```python
from build123d import *

# Parameters (mm, degrees)
SKETCH1_W           = 75
SKETCH1_H           = 85
BOSS_EXTRUDE1_DEPTH = 3
SKETCH2_R           = 2.5
BOSS_EXTRUDE2_DEPTH = 2
SKETCH3_R           = 0.75
BOSS_EXTRUDE3_DEPTH = 4
CUT_EXTRUDE1_REACH  = 58.996
CHAMFER3_SIZE       = 2.5
FILLET2_R           = 1
SKETCH5_W           = 9.85
SKETCH5_H           = 3.85
BOSS_EXTRUDE4_DEPTH = 3
FILLET3_R           = 2
SKETCH6_W           = 1.5
SKETCH6_H           = 3
CUT_EXTRUDE2_DEPTH  = 69.085465593


with BuildPart() as part:
    # Sketch1 → Boss-Extrude1 (new body)
    with BuildSketch(Plane(origin=(0, 0, 0), x_dir=(1, 0, 0), z_dir=(0, 1, 0))):
        Rectangle(SKETCH1_W, SKETCH1_H)
    extrude(amount=BOSS_EXTRUDE1_DEPTH)

    # Sketch2 → Boss-Extrude2 (add)
    with BuildSketch(Plane(origin=(0, 3, 0), x_dir=(1, 0, 0), z_dir=(0, 1, 0))):
        with Locations(Location((27.93, 36.82, 0), (0, 0, 270))):
            Circle(SKETCH2_R)
        with Locations(Location((27.93, 17.77, 0), (0, 0, 270))):
            Circle(SKETCH2_R)
        with Locations(Location((-27.93, 17.77, 0), (0, 0, 90))):
            Circle(SKETCH2_R)
        with Locations(Location((-27.93, 36.82, 0), (0, 0, 90))):
            Circle(SKETCH2_R)
        with Locations(Location((-19.05, 10.79, 0), (0, 0, 90))):
            Circle(SKETCH2_R)
        with Locations(Location((-20.32, -37.48, 0), (0, 0, 90))):
            Circle(SKETCH2_R)
        with Locations(Location((31.75, -4.45, 0), (0, 0, 270))):
            Circle(SKETCH2_R)
        with Locations(Location((31.75, -32.4, 0), (0, 0, 270))):
            Circle(SKETCH2_R)
    extrude(amount=BOSS_EXTRUDE2_DEPTH)

    # Sketch3 → Boss-Extrude3 (add)
    with BuildSketch(Plane(origin=(0, 5, 0), x_dir=(1, 0, 0), z_dir=(0, 1, 0))):
        with Locations(Location((-27.93, 36.82, 0), (0, 0, 270))):
            Circle(SKETCH3_R)
        with Locations(Location((27.93, 36.82, 0), (0, 0, 90))):
            Circle(SKETCH3_R)
        with Locations(Location((27.93, 17.77, 0), (0, 0, 270))):
            Circle(SKETCH3_R)
        with Locations(Location((-27.93, 17.77, 0), (0, 0, 90))):
            Circle(SKETCH3_R)
        with Locations(Location((-19.05, 10.79, 0), (0, 0, 270))):
            Circle(SKETCH3_R)
        with Locations(Location((31.75, -4.45, 0), (0, 0, 270))):
            Circle(SKETCH3_R)
        with Locations(Location((-20.32, -37.48, 0), (0, 0, 270))):
            Circle(SKETCH3_R)
        with Locations(Location((31.75, -32.4, 0), (0, 0, 270))):
            Circle(SKETCH3_R)
    extrude(amount=BOSS_EXTRUDE3_DEPTH)

    # Sketch4 → Cut-Extrude1 (cut, up to next)
    with BuildSketch(Plane(origin=(0, 3, 0), x_dir=(1, 0, 0), z_dir=(0, 1, 0)), mode=Mode.PRIVATE) as cut_extrude1_sk1:
        Polygon((37.5, 7.5), (32.5, 12.5), (32.5, 42.5), (37.5, 42.5), align=None)
    cut_extrude1_tool1 = extrude(cut_extrude1_sk1.sketch, amount=-CUT_EXTRUDE1_REACH, mode=Mode.PRIVATE) & part.part
    add(cut_extrude1_tool1.solids().sort_by_distance((35.064103, 3, -26.217949))[0], mode=Mode.SUBTRACT)

    # Chamfer3
    chamfer3_edges = [part.edges().sort_by_distance(p)[0] for p in [
        (37.5, 1.5, 42.5),
        (-37.5, 1.5, 42.5),
        (-37.5, 1.5, -42.5),
        (32.5, 1.5, -42.5),
    ]]
    chamfer(chamfer3_edges, length=CHAMFER3_SIZE)

    # Fillet2
    fillet2_edges = [part.edges().sort_by_distance(p)[0] for p in [
        (-37.5, 1.5, -40),
        (-37.5, 1.5, 40),
        (37.5, 1.5, 40),
        (32.5, 1.5, -40),
        (-35, 1.5, -42.5),
        (30, 1.5, -42.5),
        (37.5, 1.5, -7.5),
        (32.5, 1.5, -12.5),
        (35, 1.5, 42.5),
        (-35, 1.5, 42.5),
    ]]
    fillet(fillet2_edges, radius=FILLET2_R)

    # Sketch5 → Boss-Extrude4 (add)
    with BuildSketch(Plane.XZ):
        with Locations((10, -9.0625)):
            Rectangle(SKETCH5_W, SKETCH5_H)
        with Locations((-10, -9.0625)):
            Rectangle(SKETCH5_W, SKETCH5_H)
    extrude(amount=BOSS_EXTRUDE4_DEPTH)

    # Fillet3
    fillet3_edges = [part.edges().sort_by_distance(p)[0] for p in [
        (10, 0, -7.1375),
        (10, 0, -10.9875),
        (-10, 0, -10.9875),
        (-10, 0, -7.1375),
    ]]
    fillet(fillet3_edges, radius=FILLET3_R)

    # Sketch6 → Cut-Extrude2 (cut, through all)
    with BuildSketch(Plane.ZY.offset(14.925)):
        with Locations((-9.1375, -1.5)):
            Rectangle(SKETCH6_W, SKETCH6_H)
    extrude(amount=-CUT_EXTRUDE2_DEPTH, mode=Mode.SUBTRACT)


solid = part.part
```
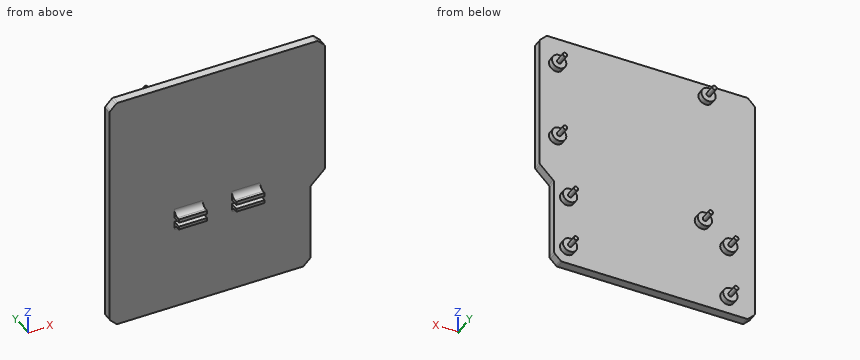
Input: part model. Units: mm. Frame: model coordinates. Give positions to 0.01 mm unless a question says otherwise; leave off trailing zeros. Order: outer loops, then holes, each group sorted by start corner. A loop starts at its lowest first (then second) coordinate and runs counter-clockwise, first axis right, second up.
1. Cut plane B-B (x = -9.5). Return loops of the section in (y, z).
Computed:
outline: (-3, -10.99) - (-2, -10.99) arc R2 cw to (0, -12.99) - (0, -42.5) - (3, -42.5) - (3, 42.5) - (0, 42.5) - (0, -5.14) arc R2 cw to (-2, -7.14) - (-3, -7.14) - (-3, -8.39) - (0, -8.39) - (0, -9.89) - (-3, -9.89) - close
2. Cut plane A-A (y = 4). Return loops of the section in (x, z).
Computed:
outline: circle Ø5 at (-27.93, -36.82); circle Ø5 at (-27.93, -17.77); circle Ø5 at (-20.32, 37.48); circle Ø5 at (-19.05, -10.79); circle Ø5 at (27.93, -36.82); circle Ø5 at (27.93, -17.77); circle Ø5 at (31.75, 4.45); circle Ø5 at (31.75, 32.4)
3. Pin query (flat end, axial travel): pin 1 Ø5 at (y, z) = (6.5, 23) entering from -X; pin 2 Ø3.5 at (y, z) = (-1.5, -12) entering from +X; pin 3 Ø6 at (x, z) = (27, 21.5) entering from -Y; pin 4 Ø1.5 at (x, z) = (-20, -11.5) entering from +Y. Return the tip coordinate at first contact, or that it passes through.
Computed:
pin 1: passes through
pin 2: stops at x = 33.9
pin 3: stops at y = 0
pin 4: stops at y = 9
4. Cut plane C-C (z = 22.5). Return loops of the section in (x, y), and give its area (3 significant figures).
Computed:
outline: (-37.5, 0) - (37.5, 0) - (37.5, 3) - (-37.5, 3) - close
area: 225 mm2
5. Line query: probe 1 along Y at (x, z) = (-11, 1.5); probe 2 along Z at (x, y) = (32, 4); probe 3 along X at (y, z) = (2.75, -10). Output: solid intervals per line, ascending.
Computed:
probe 1: y = 0 to 3
probe 2: z = 1.96 to 6.94, 29.91 to 34.89
probe 3: x = -37.5 to 35
6. Cut plane D-D (x = 21). Return loops of the section in (y, z).
Computed:
outline: (0, -42.5) - (3, -42.5) - (3, 42.5) - (0, 42.5) - close
